Job drawing, mm, ordinate dimensions from the low corner. One solid piece. Round coordinates to 2 decimals unless told otherwise and drop trailing zeros. Order: outer loops, then holes, each group sorted by start corner. A loop starts at its lowest first (then second) coordinate and runs counter-clockwise, first axis right, second up. Notation, with made-up numbers: (-35.5, 78) -> (-10.5, 78) arc R35 ccw to (-10.5, 113) -> close; hole circle Ø1 at (60, 27). An arc over 180 degrees is marked (long way). Return JSON: item names as keys, results as strings. Group by question number.
Q1. Cut at B-B (y = 2). Write the cut outline in (x, z).
Q2. Probe line 1 along Z through (x, y) = (3.55, 21.6); line 2 along Y through (x, z) = (3.55, 2.25); line 3 along X through (y, z) = (22, 3.75). List the from-to ranges inside material, lowest first.
Q3. Cut at A-A (x = 3.55). Write the cut outline in (y, z), then the cut area to 3 significant figures.
Q4. Cut at D-D (z = 3.55). Write the cut outline in (x, y), then the cut area to 3 significant figures.
Q5. Cut at C-C (y = 22.5). Write the cut outline in (x, z).
Q6. Flat gauge pin, fed straight in: pin 1 (1.4 mm diameter, centred on x = 3.55, y = 2, fed in from +Z). Where does the tip first touch, or does it go through?
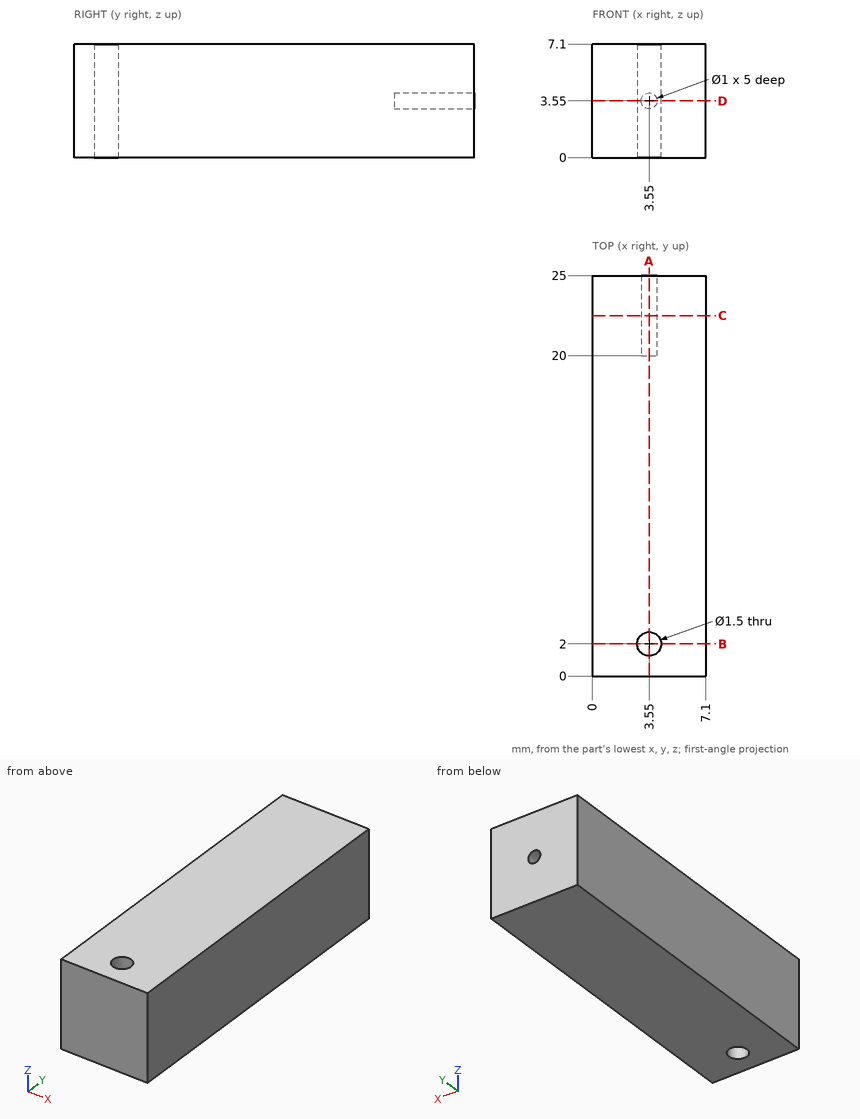
Solution:
{
 "1": {"outline": "(0, 0) -> (2.8, 0) -> (2.8, 7.1) -> (0, 7.1) -> close; (4.3, 0) -> (7.1, 0) -> (7.1, 7.1) -> (4.3, 7.1) -> close"},
 "2": {"line 1": "z = 0 to 3.05, 4.05 to 7.1", "line 2": "y = 0 to 1.25, 2.75 to 25", "line 3": "x = 0 to 3.09, 4.01 to 7.1"},
 "3": {"outline": "(0, 0) -> (1.25, 0) -> (1.25, 7.1) -> (0, 7.1) -> close; (2.75, 0) -> (25, 0) -> (25, 3.05) -> (20, 3.05) -> (20, 4.05) -> (25, 4.05) -> (25, 7.1) -> (2.75, 7.1) -> close", "area": "162 mm²"},
 "4": {"outline": "(0, 0) -> (7.1, 0) -> (7.1, 25) -> (4.05, 25) -> (4.05, 20) -> (3.05, 20) -> (3.05, 25) -> (0, 25) -> close; hole circle Ø1.5 at (3.55, 2)", "area": "171 mm²"},
 "5": {"outline": "(0, 0) -> (7.1, 0) -> (7.1, 7.1) -> (0, 7.1) -> close; hole circle Ø1 at (3.55, 3.55)"},
 "6": {"pin 1": "passes through"}
}
